Part print with two shaded views. Sizes in mm from the minimum x, y, z corner. Round coordinates to 2 decimals unless told otherwise and drop trailing zeros. Loops run counter-clockwise (first coordinate to the right, second up) from the corner with the lowest first, then second, coordinate; pieces in that order, holes last. Notation, with made-up numbers: (-32.75, 74.25) - (14.25, 74.25) arc R29 ccw to (14.25, 111.25) - close; hole circle Ø8 at (-39, 2). An arc over 180 degrees is marked (long way). Write each question's results on one line, items separated by ' | '. Start each with the question number.
(1) Cut at A-A, the plane x = 17. List the corners of the cut face in (y, z).
(2) Flat gauge pins, fed straight in: P1, Ø1, axis at y = 4.5, z = 13, coming from the -X side; P2, Ø1.3, axis at x = 5, y = 3, coming from the -Z side; P3, Ø1.8, axis at y = 3.5, z = 2.5, coming from the +X side. Where does each tip first touch, or does it go through?
(3) Drill centre lines: L1, parallel to Z at x = 103, y = 1; L2, parallel to X at y = 4.5, z = 24.5; L3, parallel to Z at x = 8, y = 5.25. Where is each one in solid material? Low to high.
(4) Cut at C-C, the plane z = 35. List the corners of the cut face in (x, y).
(5) Cut at B-B, the plane z = 27. List the corners of the cut face in (x, y).
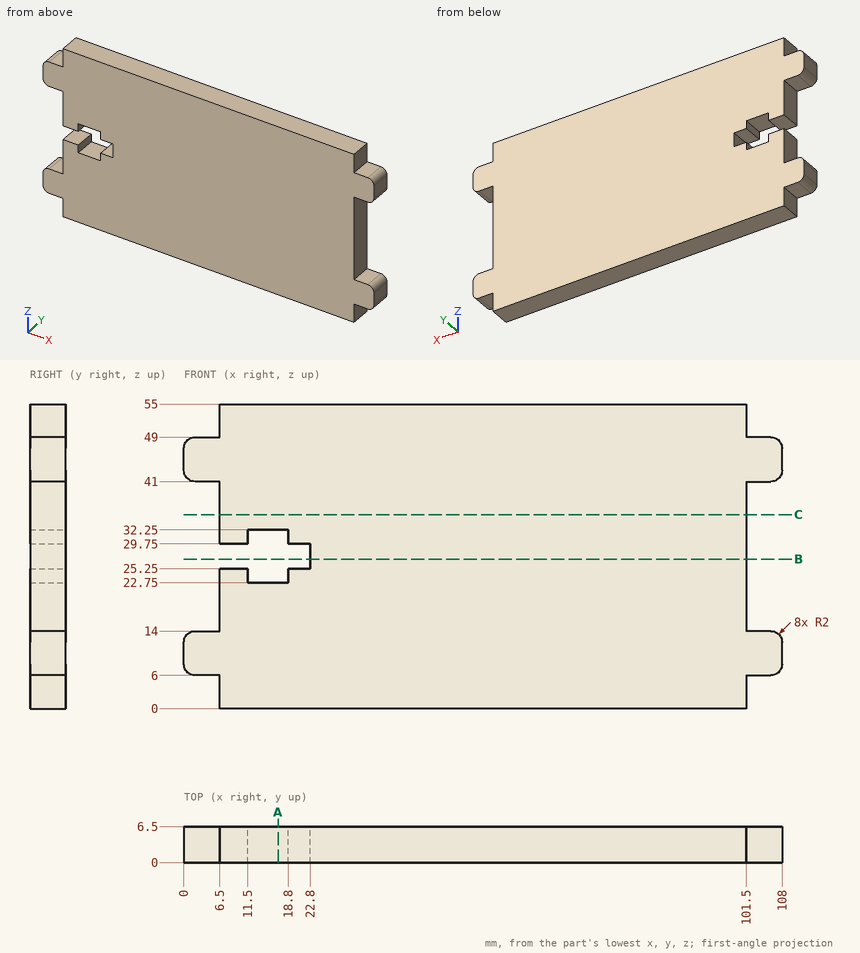
A:
1) outline: (0, 0) - (6.5, 0) - (6.5, 22.75) - (0, 22.75) - close; (0, 32.25) - (6.5, 32.25) - (6.5, 55) - (0, 55) - close
2) P1: x = 0.06 | P2: z = 6 | P3: x = 101.5
3) L1: 6 to 14, 41 to 49 | L2: 6.5 to 11.5, 18.8 to 101.5 | L3: 0 to 25.25, 29.75 to 55
4) outline: (6.5, 0) - (101.5, 0) - (101.5, 6.5) - (6.5, 6.5) - close
5) outline: (22.8, 0) - (101.5, 0) - (101.5, 6.5) - (22.8, 6.5) - close
